```python
from build123d import *

# Parameters (mm, degrees)
SKETCH1_W                = 3.530112864
SKETCH1_H                = 9.82
BOSS_EXTRUDE2_DEPTH      = 6
SKETCH1_4_W              = 6
SKETCH1_4_H              = 9.82
SKETCH1_4_W_2            = 3.530112864
BOSS_EXTRUDE3_DEPTH      = 6
BOSS_EXTRUDE4_DEPTH      = 18.469887
BOSS_EXTRUDE4_DEPTH_BACK = 31.530113


with BuildPart() as part:
    # Sketch1 → Boss-Extrude2 (new body)
    with BuildSketch(Plane(origin=(0, 0, 0), x_dir=(0, 0, -1), z_dir=(1, 0, 0))):
        with Locations((4.765056432, 4.91)):
            Rectangle(SKETCH1_W, SKETCH1_H)
        with Locations((-4.765056432, 4.91)):
            Rectangle(SKETCH1_W, SKETCH1_H)
        Polygon((6.530112864, 9.82), (6.530112864, 15.3052734), (-6.530112864, 15.3052734), (-6.530112864, 9.82), (-3, 9.82), (3, 9.82), align=None)
    extrude(amount=-BOSS_EXTRUDE2_DEPTH)

    # Sketch1<4> → Boss-Extrude3 (add)
    # profile 1 of 6: a face of its own
    with BuildSketch(Plane(origin=(0, 0, 0), x_dir=(0, 0, -1), z_dir=(1, 0, 0))):
        with Locations((0, 4.91)):
            Rectangle(SKETCH1_4_W, SKETCH1_4_H)
    # profile 2 of 6: a face of its own
    with BuildSketch(Plane(origin=(0, 0, 0), x_dir=(0, 0, -1), z_dir=(1, 0, 0))):
        Polygon((-6.530112864, 9.82), (-3, 9.82), (3, 9.82), (6.530112864, 9.82), (6.530112864, 15.3052734), (-6.530112864, 15.3052734), align=None)
    # profile 3 of 6: a face of its own
    with BuildSketch(Plane(origin=(0, 0, 0), x_dir=(0, 0, -1), z_dir=(1, 0, 0))):
        with Locations((-4.765056432, 4.91)):
            Rectangle(SKETCH1_4_W_2, SKETCH1_4_H)
    # profile 4 of 6: a face of its own
    with BuildSketch(Plane(origin=(0, 0, 0), x_dir=(0, 0, -1), z_dir=(1, 0, 0))):
        with Locations((4.765056432, 4.91)):
            Rectangle(SKETCH1_4_W_2, SKETCH1_4_H)
    # profile 5 of 6: a face of its own
    with BuildSketch(Plane(origin=(0, 0, 0), x_dir=(0, 0, -1), z_dir=(1, 0, 0))):
        with BuildLine():
            Line((-3.498344074, 24.541666174), (-6.530112864, 15.3052734))
            Line((-6.530112864, 15.3052734), (6.530112864, 15.3052734))
            Line((6.530112864, 15.3052734), (3.498344074, 24.541666174))
            Line((3.498344074, 24.541666174), (3.498344074, 43.778718631))
            Line((3.498344074, 43.778718631), (1.742466173, 54.048264378))
            ThreePointArc((1.742466173, 54.048264378), (-3.323802498, 57.355930134), (-6.240866628, 52.055131338))
            Line((-6.240866628, 52.055131338), (-3.498344074, 43.778718631))
            Line((-3.498344074, 43.778718631), (-3.498344074, 24.541666174))
        make_face()
        with BuildLine():
            Line((-4.024402568, 55.252914737), (-0.624402568, 55.252914737))
            Line((-0.624402568, 55.252914737), (-0.624402568, 53.352914737))
            ThreePointArc((-0.624402568, 53.352914737), (-1.063742396, 52.292254566), (-2.124402568, 51.852914737))
            Line((-2.124402568, 51.852914737), (-2.524402568, 51.852914737))
            ThreePointArc((-2.524402568, 51.852914737), (-3.58506274, 52.292254566), (-4.024402568, 53.352914737))
            Line((-4.024402568, 53.352914737), (-4.024402568, 55.252914737))
        make_face(mode=Mode.SUBTRACT)
    # profile 6 of 6: a face of its own
    with BuildSketch(Plane(origin=(0, 0, 0), x_dir=(0, 0, -1), z_dir=(1, 0, 0))):
        with BuildLine():
            ThreePointArc((-3.824402568, 53.352914737), (-3.443641384, 52.433675922), (-2.524402568, 52.052914737))
            Line((-2.524402568, 52.052914737), (-2.124402568, 52.052914737))
            ThreePointArc((-2.124402568, 52.052914737), (-1.205163753, 52.433675922), (-0.824402568, 53.352914737))
            Line((-0.824402568, 53.352914737), (-0.824402568, 55.052914737))
            Line((-0.824402568, 55.052914737), (-3.824402568, 55.052914737))
            Line((-3.824402568, 55.052914737), (-3.824402568, 53.352914737))
        make_face()
    extrude(amount=BOSS_EXTRUDE3_DEPTH)


with BuildPart() as boss_extrude3_kept_piece:
    # of the separate pieces the step leaves, the one the design keeps (boss_extrude3_pieces_kept)
    add(part.part.solids().sort_by_distance((6, 0, -6.530112864))[0])

    # Sketch4 → Boss-Extrude4 (add, two sides: drawn at the far end of the back side and taken through both)
    with BuildSketch(Plane.XY.offset(6.530112864).offset(-BOSS_EXTRUDE4_DEPTH_BACK)):
        with BuildLine():
            Line((6, 0), (0.292808536, 0))
            Line((0.292808536, 0), (0.292808536, 1.707191464))
            ThreePointArc((0.292808536, 1.707191464), (1.464381411, 4.535618589), (4.292808536, 5.707191464))
            Line((4.292808536, 5.707191464), (6, 5.707191464))
            Line((6, 5.707191464), (6, 0))
        make_face()
    extrude(amount=BOSS_EXTRUDE4_DEPTH + BOSS_EXTRUDE4_DEPTH_BACK)


solid = boss_extrude3_kept_piece.part
```
Check sheet for the modelled part. Datum: model origin and axes. Units: mm. A direction names the side the tool comes from. Round coordinates to 2 decimals unless told otherwise and drop trailing zeros. Order: outer loops, then holes, each group sorted by start corner. A loop starts at its lowest first (then second) coordinate and runs counter-clockwise, first axis right, second up. Notation, with made-up numbers: (40.5, 73.25) - (99.5, 73.25) arc R27 cw to (99.5, 101.25) - close; hole circle Ø7 at (65.25, -23.75). An arc over 180 degrees is marked (long way). Write item = value, one per line.
Q1. Section check B-B (z = 16). Record the boundary of the cut face in (x, y).
Computed:
outline = (0.29, 0) - (6, 0) - (6, 5.71) - (4.29, 5.71) arc R4 ccw to (0.29, 1.71) - close
Q2. Thickness scan on line 1 along Z through (x, y) = (-3.5, 11); line 2 along Y through (x, z) = (5.25, -22); line 3 along X through (y, z) = (40.5, 0). Record the ranges inside material, lowest first.
Computed:
line_1 = -6.53 to 6.53
line_2 = 0 to 5.71
line_3 = 0 to 6
Q3. Tool access check on faces 1 (the face through (0.293, 1, -16)), 2 (the face through (3, 55.253, 2)), 3 (the face through (-3, 9.82, 0)). Record the directions out of +Z, -Z, +X, -X, +Y, -Y that give a thin tool (end or side, any length) a straight path to the whole face; none if there is none.
Computed:
face_1 = -Z, -X, +Y, -Y
face_2 = +X, -X
face_3 = -X, -Y
Q4. Section check C-C (y = 7). Record the boundary of the cut face in (x, z).
Computed:
outline = (-6, -6.53) - (6, -6.53) - (6, 6.53) - (-6, 6.53) - (-6, 3) - (0, 3) - (0, -3) - (-6, -3) - close
Q5. Draft check along Z on faces 4 (the face through (-3, 15.305, 0)), 5 (the face through (0, 9, 6.53)), 6 (the face through (2.96, 52.28, 3.57)). Enter one of: pulls with the +Z half, pulls with the -Z half, needs draft (parallel to the pull), parting line crosses it, or undercut.
Computed:
face_4 = needs draft
face_5 = pulls with the +Z half
face_6 = undercut
Q6. Go/stop test with flat-tipped pins: pin 1 (14.5 mm diameter, centred on y = 32, z = -1, fed in from -X); pin 2 (3.5 mm diameter, centred on x = -0.5, y = 6.5, fed in from +Z); pin 3 (5 mm diameter, centred on x = 2.5, y = 38, fed in from -Z); pin 4 (1.5 mm diameter, centred on y = 9, z = -7.5, fed in from +X). Record where each tip stops, or that it passes through.
Computed:
pin_1 = 0
pin_2 = 6.53
pin_3 = -3.5
pin_4 = through
Q7. Section check D-D (x = 2.75). Record the boundary of the cut face in (y, z).
Computed:
outline = (0, -25) - (5.4, -25) - (5.4, -6.53) - (15.31, -6.53) - (24.54, -3.5) - (43.78, -3.5) - (54.05, -1.74) arc R4.13 ccw (long way) to (52.06, 6.24) - (43.78, 3.5) - (24.54, 3.5) - (15.31, 6.53) - (5.4, 6.53) - (5.4, 25) - (0, 25) - close; hole (51.85, 2.12) arc R1.5 ccw to (53.35, 0.62) - (55.25, 0.62) - (55.25, 4.02) - (53.35, 4.02) arc R1.5 ccw to (51.85, 2.52) - close
Q8. Section check A-A (x = -4). Record the boundary of the cut face in (y, z).
Computed:
outline = (0, -6.53) - (15.31, -6.53) - (15.31, 6.53) - (0, 6.53) - (0, 3) - (9.82, 3) - (9.82, -3) - (0, -3) - close
